from build123d import *

# Parameters (mm, degrees)
SKETCH_3_W               = 86
SKETCH_3_H               = 15
EXTRUDE_1_DEPTH          = 2
EXTRUDE_START            = -3
EXTRUDE_2_DEPTH          = 9
EXTRUDE_START_2          = 2
EXTRUDE_3_DEPTH          = 2
CUT_EXTRUDE_1_REACH      = 87.235
CUT_EXTRUDE_1_END_RADIUS = 68.229392493
SKETCH_7_W               = 75
SKETCH_7_H               = 9
SKETCH_8_R               = 1.6
CUT_EXTRUDE_2_DEPTH      = 86.234584505
CUT_EXTRUDE_START        = -3
SKETCH_9_R               = 3
CUT_EXTRUDE_3_DEPTH      = 83.234584523


with BuildPart() as part:
    # 草图3 → 凸台-拉伸1 (new body)
    with BuildSketch(Plane(origin=(0, 0, 0), x_dir=(1, 0, 0), z_dir=(0, 1, 0))):
        with Locations((40, 4.5)):
            Rectangle(SKETCH_3_W, SKETCH_3_H)
    extrude(amount=EXTRUDE_1_DEPTH)

    # 草图5 → 凸台-拉伸2 (add)
    with BuildSketch(Plane.XY.offset(3).offset(EXTRUDE_START)):
        with BuildLine():
            Line((2.5, 0), (-1.026425264, 0))
            ThreePointArc((-1.026425264, 0), (40, -13.229392493), (81.026425264, 0))
            Line((81.026425264, 0), (77.5, 0))
            ThreePointArc((77.5, 0), (40, -11.229392493), (2.5, 0))
        make_face()
    extrude(amount=-EXTRUDE_2_DEPTH)

    # 草图6 → 凸台-拉伸3 (add)
    with BuildSketch(Plane.XY.offset(EXTRUDE_START_2)):
        with BuildLine():
            Line((-1.026425264, 0), (81.026425264, 0))
            ThreePointArc((81.026425264, 0), (40, -13.229392493), (-1.026425264, 0))
        make_face()
    extrude_3 = extrude(amount=-EXTRUDE_3_DEPTH)

    # 镜向1: 凸台-拉伸3 across plane
    add(extrude_3.mirror(Plane.XY.offset(-4.5)))

    # 切除-拉伸1: up to this cylinder (the profile starts inside it)
    cut_extrude_1_end = Plane(origin=(40, 57, -4.5), z_dir=(0, 0, 1)) * Cylinder(CUT_EXTRUDE_1_END_RADIUS, 311.928784987, mode=Mode.PRIVATE)
    # 草图7 → 切除-拉伸1 (cut, up to the surface)
    with BuildSketch(Plane(origin=(0, 2, 0), x_dir=(1, 0, 0), z_dir=(0, 1, 0)), mode=Mode.PRIVATE) as cut_extrude_1_sk1:
        with Locations((40, 4.5)):
            Rectangle(SKETCH_7_W, SKETCH_7_H)
    cut_extrude_1_tool1 = extrude(cut_extrude_1_sk1.sketch, amount=-CUT_EXTRUDE_1_REACH, mode=Mode.PRIVATE) & cut_extrude_1_end
    add(cut_extrude_1_tool1.solids().sort_by_distance((40, 2, -4.5))[0], mode=Mode.SUBTRACT)

    # 草图8 → 切除-拉伸2 (cut, through all)
    with BuildSketch(Plane(origin=(0, 2, 0), x_dir=(1, 0, 0), z_dir=(0, 1, 0))):
        with Locations(Location((80, 0, 0), (0, 0, 270))):
            Circle(SKETCH_8_R)
        with Locations(Location((80, 9, 0), (0, 0, 270))):
            Circle(SKETCH_8_R)
        with Locations(Location((0, 0, 0), (0, 0, 270))):
            Circle(SKETCH_8_R)
        with Locations(Location((0, 9, 0), (0, 0, 270))):
            Circle(SKETCH_8_R)
    extrude(amount=-CUT_EXTRUDE_2_DEPTH, mode=Mode.SUBTRACT)

    # 草图9 → 切除-拉伸3 (cut, through all)
    with BuildSketch(Plane(origin=(0, 2, 0), x_dir=(1, 0, 0), z_dir=(0, 1, 0)).offset(CUT_EXTRUDE_START)):
        with Locations((0, 9)):
            Circle(SKETCH_9_R)
        Circle(SKETCH_9_R)
        with Locations((80, 0)):
            Circle(SKETCH_9_R)
        with Locations((80, 9)):
            Circle(SKETCH_9_R)
    extrude(amount=-CUT_EXTRUDE_3_DEPTH, mode=Mode.SUBTRACT)


solid = part.part
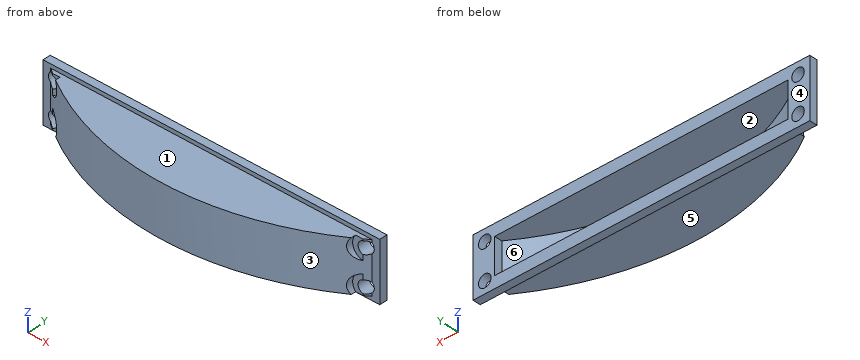
For this review, take the finished solid that the model builds, in its own axes (mm). Face numbers are marked on the shaded views. A direction names the side the tool comes from. Give positions to 0.01 mm unless a question says otherwise; leave off trailing zeros. Loops run counter-clockwise (first coordinate to the right, second up) from the corner with the lowest first, then second, coordinate; pieces in that order, holes last. Notation, with made-up numbers: M 35,71 L 78,71 A20 cw 78,83 Z; hole C 26.25,69.25 d4. An arc over 180 degrees is marked long. Answer as a JSON object with one key per item and string values. Group by question number.
Q1. Mouldability with a two-part tool opening along X and no side actions: class the marked faces 1, 2 and 3 as +X half, -X half, draft (parallel to the pull), parting line (faces both ways), or undercut.
Q2. Tool access review of the marked faces 4, 5 and 6: name each direction out of +Z, -Z, +X, -X, +Y, -Y from which nothing blocks a thin tool from reaching the whole face with its end or side.
Q3. Insertion check: P1, Ø5, axis at x = 6, z = -1.5, coming from the -Y side; P2, Ø5, axis at x = 59.5, y = -7, coming from the +Z side; P3, Ø2, axis at x = 1.5, z = 0.5, coming from the -Y side. Each pin has a flat end and moves straight along its axis. Give the tip position at first contact, or say it passes through.
Q4. Add section B-B on z = -3.75. Give the boundary of the cut face in (x, y).
Q5. Add section D-D on x = 67.5. Give the boundary of the cut face in (y, z), and give its area (3 significant figures).
Q6. Add section A-A on y = -6. Give the boundary of the cut face in (x, z), and give its area (3 significant figures).
Q7. Add section C-C on x = 20.5. Give the boundary of the cut face in (y, z).
Q8. For probe 1 along Z at (x, y) = (80, -0.2); probe 2 along Z at (x, y) = (0, 0.65); probe 3 along Z at (x, y) = (42, -1), list the stretches that pass through material, from the lowest coordinate up. Write a range as [from, to].
Checked values:
{
 "1": {"face 1": "draft", "face 2": "undercut", "face 3": "parting line"},
 "2": {"face 4": "+Z, -Z, +X, -X, +Y", "face 5": "-Z, +X, -X, -Y", "face 6": "+Y"},
 "3": {"P1": "y = -5.77", "P2": "z = 2", "P3": "y = -1"},
 "4": {"outline": "M -3,0 L -1.03,0 A70.23 ccw 81.03,0 L 83,0 L 83,2 L 77.5,2 L 77.5,0 A68.23 cw 2.5,0 L 2.5,2 L -3,2 Z"},
 "5": {"outline": "M -7.62,-11 L 0,-11 L 0,-12 L 2,-12 L 2,-9 L -5.44,-9 L -5.44,0 L 2,0 L 2,3 L 0,3 L 0,2 L -7.62,2 Z", "area": "62.1 mm²"},
 "6": {"outline": "M 8.97,-11 L 71.03,-11 L 71.03,2 L 8.97,2 Z; hole M 13.8,-9 L 66.2,-9 L 66.2,0 L 13.8,0 Z", "area": "335 mm²"},
 "7": {"outline": "M -10.47,-11 L 0,-11 L 0,-12 L 2,-12 L 2,-9 L -8.38,-9 L -8.38,0 L 2,0 L 2,3 L 0,3 L 0,2 L -10.47,2 Z"},
 "8": {"probe 1": "[-11, -10.6], [-7.4, -1.6], [1.6, 2]", "probe 2": "[-12, -10.6], [-7.4, -1.6], [1.6, 3]", "probe 3": "[-11, -9], [0, 2]"}
}
